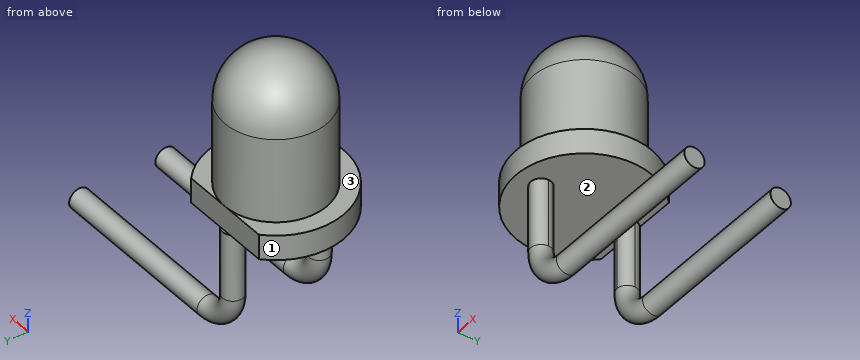
from build123d import *

# Parameters (mm, degrees)
F3_DEPTH  = 25
F5_DEPTH  = 2
F5_FACE_R = 0.3
F6_R      = 0.3
F7_ANGLE  = 90
F8_R      = 0.3
F7_FACE_R = 0.3
F9_DEPTH  = 5


with BuildPart() as f1:
    # F0 (on Front) → F1 (revolve)
    with BuildSketch(Plane.XZ):
        with BuildLine():
            Line((0, 4), (0, 0))
            Line((0, 0), (0, -0.7406895747))
            Line((0, -0.7406895747), (2, -0.7406895747))
            Line((2, -0.7406895747), (2, 0))
            Line((2, 0), (1.5, 0))
            Line((1.5, 0), (1.5, 2.5))
            ThreePointArc((1.5, 2.5), (1.0606601718, 3.5606601718), (0, 4))
        make_face()
    revolve(axis=Axis((0, 0, 2), (0, 0, 1)))

    # F2 (on face) → F3 (cut)
    with BuildSketch(Plane(origin=(0, 0, -0.7406895747), x_dir=(1, 0, 0), z_dir=(0, 0, -1))):
        with BuildLine():
            Line((1.3228756555, -1.5), (-1.3228756555, -1.5))
            ThreePointArc((-1.3228756555, -1.5), (0, -2), (1.3228756555, -1.5))
        make_face()
    extrude(amount=-F3_DEPTH, mode=Mode.SUBTRACT)

    # F4 (on face) → F5 (join)
    with BuildSketch(Plane(origin=(0, 0, -0.7406895747), x_dir=(1, 0, 0), z_dir=(0, 0, -1))):
        with BuildLine():
            ThreePointArc((0, 0.97), (0.2121320344, 1.0578679656), (0.3, 1.27))
            ThreePointArc((0.3, 1.27), (-0.2121320344, 1.4821320344), (0, 0.97))
        make_face()
        with BuildLine():
            ThreePointArc((0.3, -1.27), (0.2121320344, -1.0578679656), (0, -0.97))
            ThreePointArc((0, -0.97), (-0.2121320344, -1.4821320344), (0.3, -1.27))
        make_face()
    extrude(amount=F5_DEPTH)

    # F5_face (on face) + F6 (on face) → F7 (revolve)
    with BuildSketch(Plane(origin=(0, 1.27, -2.7406895747), x_dir=(1, 0, 0), z_dir=(0, 0, -1))):
        with Locations((0, 2.54)):
            Circle(F5_FACE_R)
    with BuildSketch(Plane(origin=(0, 0, -2.7406895747), x_dir=(1, 0, 0), z_dir=(0, 0, -1))):
        with Locations((0, -1.27)):
            Circle(F6_R)
    revolve(axis=Axis((1, 0.2732329885, -2.7406895747), (0, -1, 0)), revolution_arc=F7_ANGLE)

    # F8 (on face) + F7_face (on face) → F9 (join)
    with BuildSketch(Plane.YZ.offset(1)):
        with Locations((-1.27, -3.7406895747)):
            Circle(F8_R)
    with BuildSketch(Plane(origin=(1, -1.27, -3.7406895747), x_dir=(0, 1, 0), z_dir=(1, 0, 0))):
        with Locations((2.54, 0)):
            Circle(F7_FACE_R)
    extrude(amount=F9_DEPTH)


solid = f1.part
Input: part model. Units: mm. Frame: model coordinates. Face numbers are marked on the shaded views. Coordinates: 2 decimals unless noted, no trailing zeros. Loops run counter-clockwise (first coordinate to the right, second up) from the corner with the lowest first, then second, coordinate; pieces in that order, holes last. Notation, with made-up numbers: (69, 73.5) -> (124, 73.5) arc R19 cw to (124, 92.5) -> close; hole circle Ø3 at (54.25, 32.25). An arc over 180 degrees is marked (long way). One line per item, written item: value.
(1) Cut plane B-B (x = 2.25). Output: boundary loops of the cut face in (y, z), then the cut area to 3 significant figures.
Answer below:
outline: circle Ø0.6 at (-1.27, -3.74); circle Ø0.6 at (1.27, -3.74)
area: 0.565 mm2
(2) Cut plane C-C (z = -2). Output: boundary loops of the cut face in (x, y).
Answer below:
outline: circle Ø0.6 at (0, -1.27); circle Ø0.6 at (0, 1.27)
(3) Cut plane A-A (y = 0). Output: boundary loops of the cut face in (x, z).
Answer below:
outline: (-2, -0.74) -> (2, -0.74) -> (2, 0) -> (1.5, 0) -> (1.5, 2.5) arc R1.5 ccw to (-1.5, 2.5) -> (-1.5, 0) -> (-2, 0) -> close
(4) Draft query along Z for the marked faces 1, 2 and 3. Return one class per face: pulls with the +Z half, pulls with the -Z half, needs draft (parallel to the pull), parting line crosses it, or undercut.
Answer below:
face 1: needs draft
face 2: undercut
face 3: pulls with the +Z half
(5) Ray query, line 1 along Z through (x, y) = (-1.5, 0.7); line 2 along Y through (x, z) = (0, 0.75); line 3 along Z through (x, y) = (-1, 0.85). Return the intervals inside material, ascending.
Answer below:
line 1: z = -0.74 to 0
line 2: y = -1.5 to 1.5
line 3: z = -0.74 to 3.23
(6) Pin query (flat end, axial travel): pin 1 Ø1.5 at (x, y) = (2, -0.5) entering from +Z; pin 2 Ø0.6 at (x, z) = (0, 0) entering from +Y; pin 3 Ø1 at (x, z) = (5, -2) entering from -Y. Return the tip coordinate at first contact, or that it passes through.
Answer below:
pin 1: stops at z = 3.23
pin 2: stops at y = 1.5
pin 3: passes through
(7) Cut plane D-D (z = 2). Output: boundary loops of the cut face in (x, y), then the cut area to 3 significant figures.
Answer below:
outline: circle Ø3 at (0, 0)
area: 7.07 mm2
